from build123d import *

# Parameters (mm, degrees)
PAD_DEPTH     = 7.5
SKETCH002_W   = 34
SKETCH002_H   = 6.8
PAD001_DEPTH  = 0.6
SKETCH001_W   = 35.08
SKETCH001_H   = 7.18
PAD002_DEPTH  = 14
PAD003_DEPTH  = 0.5
PAD004_DEPTH  = 0.5
SKETCH005_W   = 35.08
SKETCH005_H   = 7.18
SKETCH005_W_2 = 15.99
SKETCH005_H_2 = 4.8
PAD005_DEPTH  = 1
POCKET_DEPTH  = 16.5


with BuildPart() as part:
    # Sketch → Pad (new body)
    with BuildSketch(Plane.XY):
        Polygon((-20.01, 4), (-3.25, 4), (-3.25, 5), (3.25, 5), (3.25, 4), (20.01, 4), (20.01, -4), (-20.01, -4), align=None)
        Polygon((-19.01, 3), (-2.25, 3), (-2.25, 4), (2.25, 4), (2.25, 3), (19.01, 3), (19.01, -3), (-19.01, -3), align=None, mode=Mode.SUBTRACT)
    extrude(amount=-PAD_DEPTH)

    # Sketch002 → Pad001 (join)
    with BuildSketch(Plane.XY):
        Polygon((-20.01, 4), (-20.01, -4), (20.01, -4), (20.01, 4), (3.25, 4), (3.25, 5), (-3.25, 5), (-3.25, 4), align=None)
        Rectangle(SKETCH002_W, SKETCH002_H, mode=Mode.SUBTRACT)
    extrude(amount=PAD001_DEPTH)

    # Sketch001 → Pad002 (join)
    with BuildSketch(Plane.XY):
        Rectangle(SKETCH001_W, SKETCH001_H)
        with BuildLine():
            Line((16.54, 2.59), (16.54, -2.59))
            Line((16.54, -2.59), (8.82, -2.59))
            Line((8.82, -0.5), (8.82, -2.59))
            ThreePointArc((8.82, -0.5), (8.673553, -0.146447), (8.32, 0))
            Line((6.92, 0), (8.32, 0))
            ThreePointArc((6.92, 0), (6.566447, -0.146447), (6.42, -0.5))
            Line((6.42, -2.59), (6.42, -0.5))
            Line((6.42, -2.59), (-11.46, -2.59))
            Line((-11.46, -2.59), (-11.46, 2.59))
            Line((-11.46, 2.59), (8.96, 2.59))
            Line((8.96, 0.5), (8.96, 2.59))
            ThreePointArc((8.96, 0.5), (9.106447, 0.146447), (9.46, 0))
            Line((10.86, 0), (9.46, 0))
            ThreePointArc((10.86, 0), (11.213553, 0.146447), (11.36, 0.5))
            Line((11.36, 2.59), (11.36, 0.5))
            Line((11.36, 2.59), (16.54, 2.59))
        make_face(mode=Mode.SUBTRACT)
    extrude(amount=PAD002_DEPTH)

    # Sketch003 (on Face1 of Pad) → Pad003 (join)
    with BuildSketch(Plane(origin=(0, 4, 0), x_dir=(-1, 0, 0), z_dir=(0, 1, 0))):
        Polygon((15, -6), (16.5, -1.5), (13.5, -1.5), align=None)
    extrude(amount=PAD003_DEPTH)

    # Sketch004 (on Face33 of Pad003) → Pad004 (join)
    with BuildSketch(Plane.XZ.offset(3.59)):
        Polygon((16.568533, 6.35), (15.24, 12.7), (14.028533, 6.35), align=None)
    extrude(amount=PAD004_DEPTH)

    # Sketch005 → Pad005 (join)
    with BuildSketch(Plane.XY.offset(14)):
        Rectangle(SKETCH005_W, SKETCH005_H)
        with Locations((-8.445, 0)):
            Rectangle(SKETCH005_W_2, SKETCH005_H_2, mode=Mode.SUBTRACT)
        with Locations((8.445, 0)):
            Rectangle(SKETCH005_W_2, SKETCH005_H_2, mode=Mode.SUBTRACT)
    extrude(amount=PAD005_DEPTH)

    # Sketch006 → Pocket (cut, symmetric)
    with BuildSketch(Plane.YZ):
        Polygon((-3, 0), (-3, -1), (3, -1), (3, 0), (0, 3), align=None)
    extrude(amount=POCKET_DEPTH, both=True, mode=Mode.SUBTRACT)


solid = part.part
Geometry check sheet. Reference: the model listing, model coordinates, mm. A direction names the side the tool comes from. Give positions to 0.01 mm unless a question says otherwise; leave off trailing zeros. Order: outer loops, then holes, each group sorted by start corner. A loop starts at its lowest first (then second) coordinate and runs counter-clockwise, first axis right, second up.
1. Sectioned sample at A-A (z = -4.5). Record the boundary of the cut face in (x, y), then the cut area to 3 significant figures.
Completed:
outline: (-20.01, -4) - (20.01, -4) - (20.01, 4) - (3.25, 4) - (3.25, 5) - (-3.25, 5) - (-3.25, 4) - (-14.5, 4) - (-14.5, 4.5) - (-15.5, 4.5) - (-15.5, 4) - (-20.01, 4) - close; hole (-19.01, -3) - (19.01, -3) - (19.01, 3) - (2.25, 3) - (2.25, 4) - (-2.25, 4) - (-2.25, 3) - (-19.01, 3) - close
area: 94.5 mm2
2. Depth check by flat-ended pin: pin 1 (3.5 mm diameter, centred on y = -1, z = 6, fed in from -X); pin 2 (0.8 mm diameter, centred on y = 1, z = 14.5, fed in from +X); pin 3 (1.5 mm diameter, centred on x = -14.5, z = -4.5, fed in from +Y). Enter the tip coordinate at first touch or a pass-through.
Completed:
pin 1: stops at x = -17.54
pin 2: stops at x = 17.54
pin 3: stops at y = 4.5
3. Access from +Z, -Z, +X, -X, +Y, -Y to the whole of each face (thin tool, end or side, straight path). Record for faces 4 (the face through (8, -1, 14)), 5 (the face through (-14.24, 4.25, -3.72)), 6 (the face through (17.54, 0, 8)), 7 (the face through (13, -2.59, 7)), 8 (the face through (-3.25, 4.5, -3.5)).
Completed:
face 4: +Z
face 5: -Z, +Y
face 6: +Z, +X, +Y, -Y
face 7: -Z
face 8: +Z, -Z, +Y
4. Draft check along Y on faces 1 (the face through (-2.4, 2.8, 0.2)), 2 (the face through (12, 4, -4)), 3 (the face through (-17.54, 0, 8)). Enter one of: pulls with the +Y half, pulls with the -Y half, needs draft (parallel to the pull), parting line crosses it, or undercut.
Completed:
face 1: undercut
face 2: pulls with the +Y half
face 3: needs draft
5. Sectioned sample at C-C (y = -1.75). State how many separate pieces and enclosed holes the cut face has, then the cut area to 3 significant figures.
Completed:
separate pieces: 4
enclosed holes: 0
area: 144 mm2
6. Sectioned sample at B-B (x = 13). Record the boundary of the cut face in (y, z), then the cut area to 3 significant figures.
Completed:
outline: (-4, -7.5) - (-3, -7.5) - (-3, 0) - (-2.59, 0.41) - (-2.59, 14) - (-2.4, 14) - (-2.4, 15) - (-3.59, 15) - (-3.59, 0.6) - (-4, 0.6) - close; (2.4, 14) - (2.59, 14) - (2.59, 0.41) - (3, 0) - (3, -7.5) - (4, -7.5) - (4, 0.6) - (3.59, 0.6) - (3.59, 15) - (2.4, 15) - close
area: 45.7 mm2
7. Scan lines: line 1 (X direction, y = -1.75, z = 5); line 2 (Y direction, x = -7, z = 2.75); line 3 (X direction, y = 1, z = -3). Record each from-to range of solid material in increasing order.
Completed:
line 1: x = -17.54 to -11.46, 6.42 to 8.82, 16.54 to 17.54
line 2: y = -3.59 to -2.59, 2.59 to 3.59
line 3: x = -20.01 to -19.01, 19.01 to 20.01
